Check sheet for the drawn part. Datum: minimum x, y, z corner. Units: mm. Coordinates: 2 decimals unless noted, no trailing zeros. Write each loop counter-clockwise with the first axis right and the second up, starting at its lowest first coordinate (ties: lowest second). Pieces come first, ordered by that corner, then holes. Notation, with made-up numbers: (64, 51.5) -> (111, 51.5) arc R26 cw to (111, 65.5) -> close; hole circle Ø9 at (35.25, 86). An arc over 180 degrees is marked (long way). Write each question's results on one line, items separated by ' | '. Start each with the question number.
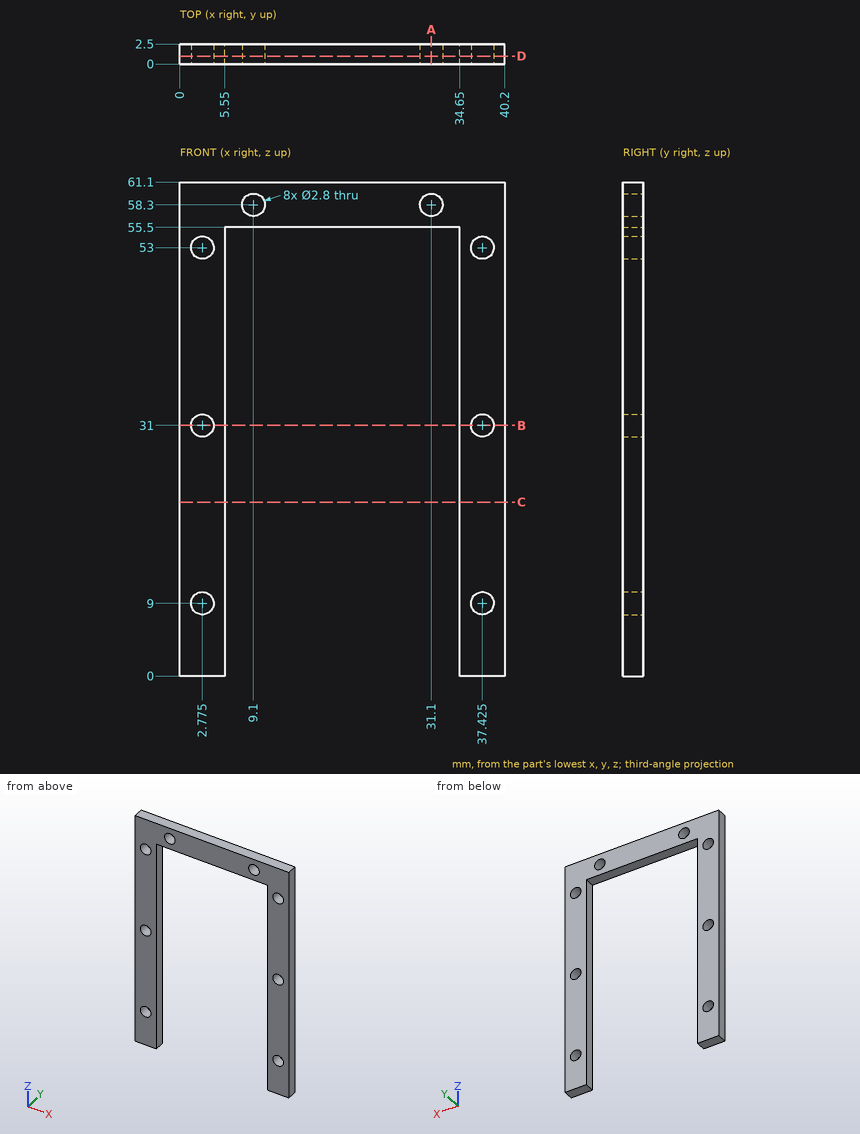
1. Depth check by flat-ended pin: pin 1 Ø2 at (x, z) = (2.775, 9) entering from -Y; pin 2 Ø4.5 at (x, z) = (37.425, 31) entering from -Y; pin 3 Ø0.8 at (x, y) = (27, 1.5) entering from -Z. Enter the tip coordinate at first touch or a pass-through.
2. Sectioned sample at C-C on z = 21.5. Record the cut outline in (x, y), plus the area to 4 significant figures.
3. Material ranges on probe 1 along X at (y, z) = (1, 31) (3 decimals); probe 2 along X at (y, z) = (1.9, 5); probe 3 along X at (y, z) = (1.35, 58.3), recorded low to high. Write a range as from..to.
4. Sectioned sample at D-D on y = 1. State how many separate pieces and enclosed holes the cut face has, plus the area to 3 significant figures.
5. Sectioned sample at B-B on z = 31. Record the cut outline in (x, y) (3 decimals).
6. Sectioned sample at A-A on x = 31.1. Record the cut outline in (y, z), plus the area to 3 significant figures.
Computed values:
1) pin 1: passes through | pin 2: stops at y = 0 | pin 3: stops at z = 55.5
2) outline: (0, 0) -> (5.55, 0) -> (5.55, 2.5) -> (0, 2.5) -> close; (34.65, 0) -> (40.2, 0) -> (40.2, 2.5) -> (34.65, 2.5) -> close | area: 27.75 mm^2
3) probe 1: x = 0..1.375, 4.175..5.55, 34.65..36.025, 38.825..40.2 | probe 2: x = 0..5.55, 34.65..40.2 | probe 3: x = 0..7.7, 10.5..29.7, 32.5..40.2
4) separate pieces: 1 | enclosed holes: 8 | area: 792 mm^2
5) outline: (0, 0) -> (1.375, 0) -> (1.375, 2.5) -> (0, 2.5) -> close; (4.175, 0) -> (5.55, 0) -> (5.55, 2.5) -> (4.175, 2.5) -> close; (34.65, 0) -> (36.025, 0) -> (36.025, 2.5) -> (34.65, 2.5) -> close; (38.825, 0) -> (40.2, 0) -> (40.2, 2.5) -> (38.825, 2.5) -> close
6) outline: (0, 55.5) -> (2.5, 55.5) -> (2.5, 56.9) -> (0, 56.9) -> close; (0, 59.7) -> (2.5, 59.7) -> (2.5, 61.1) -> (0, 61.1) -> close | area: 7.00 mm^2
